from build123d import *

# Parameters (mm, degrees)
CROQUIS1_W              = 3
CROQUIS1_H              = 15
CROQUIS1_R              = 1.25
SALIENTE_EXTRUIR1_DEPTH = 3
CROQUIS2_W              = 3
CROQUIS2_H              = 15
CORTAR_EXTRUIR1_DEPTH   = 3
CROQUIS3_W              = 10
CROQUIS3_H              = 3
SALIENTE_EXTRUIR2_DEPTH = 3
CROQUIS4_W              = 12
CROQUIS4_H              = 18.363871442
CORTAR_EXTRUIR2_DEPTH   = 3


with BuildPart() as part:
    # Croquis1 → Saliente-Extruir1 (new body)
    with BuildSketch(Plane.XY):
        with BuildLine():
            Line((103, 21.25), (103, 30))
            Line((103, 30), (69.2, 30))
            Line((69.2, 30), (69.2, 22))
            Line((69.2, 22), (71.35, 22))
            Line((71.35, 22), (71.35, 19))
            Line((71.35, 19), (69.2, 19))
            Line((69.2, 19), (69.2, 15))
            Line((69.2, 15), (66.5, 15))
            Line((66.5, 15), (66.5, 19))
            Line((66.5, 19), (64.35, 19))
            Line((64.35, 19), (64.35, 22))
            Line((64.35, 22), (66.5, 22))
            Line((66.5, 22), (66.5, 30))
            Line((66.5, 30), (36.5, 30))
            Line((36.5, 30), (36.5, 22))
            Line((36.5, 22), (38.65, 22))
            Line((38.65, 22), (38.65, 19))
            Line((38.65, 19), (36.5, 19))
            Line((36.5, 19), (36.5, 15))
            Line((36.5, 15), (33.8, 15))
            Line((33.8, 15), (33.8, 19))
            Line((33.8, 19), (31.65, 19))
            Line((31.65, 19), (31.65, 22))
            Line((31.65, 22), (33.8, 22))
            Line((33.8, 22), (33.8, 30))
            Line((33.8, 30), (0, 30))
            Line((0, 30), (0, 21.25))
            Line((0, 21.25), (1.5, 21.25))
            ThreePointArc((1.5, 21.25), (2.75, 20), (1.5, 18.75))
            Line((1.5, 18.75), (0, 18.75))
            Line((0, 18.75), (0, 0))
            Line((0, 0), (0, -10))
            Line((0, -10), (3, -10))
            Line((3, -10), (3, -20))
            Line((3, -20), (0, -20))
            Line((0, -20), (0, -35))
            Line((0, -35), (3, -35))
            Line((3, -35), (3, -50))
            Line((3, -50), (0, -50))
            Line((0, -50), (0, -65))
            Line((0, -65), (3, -65))
            Line((3, -65), (3, -80))
            Line((3, -80), (0, -80))
            Line((0, -80), (0, -92))
            Line((0, -92), (6.427876097, -99.660444431))
            Line((6.427876097, -99.660444431), (8.726009426, -97.732081602))
            Line((8.726009426, -97.732081602), (15.153885523, -105.392526033))
            Line((15.153885523, -105.392526033), (12.855752194, -107.320888862))
            Line((12.855752194, -107.320888862), (19.283628291, -114.981333294))
            Line((19.283628291, -114.981333294), (80.56718374, -63.558324519))
            Line((80.56718374, -63.558324519), (80.56718374, -50))
            Line((80.56718374, -50), (77.56718374, -50))
            Line((77.56718374, -50), (77.56718374, -35))
            Line((77.56718374, -35), (103, -35))
            Line((103, -35), (103, -16.25))
            Line((103, -16.25), (101.5, -16.25))
            ThreePointArc((101.5, -16.25), (100.25, -15), (101.5, -13.75))
            Line((101.5, -13.75), (103, -13.75))
            Line((103, -13.75), (103, 18.75))
            Line((103, 18.75), (101.5, 18.75))
            ThreePointArc((101.5, 18.75), (100.25, 20), (101.5, 21.25))
            Line((101.5, 21.25), (103, 21.25))
        make_face()
        with Locations((79.06718374, 2.5)):
            Rectangle(CROQUIS1_W, CROQUIS1_H, mode=Mode.SUBTRACT)
        with Locations((79.06718374, 20)):
            Circle(CROQUIS1_R, mode=Mode.SUBTRACT)
    extrude(amount=SALIENTE_EXTRUIR1_DEPTH)

    # Croquis2 → Cortar-Extruir1 (cut)
    with BuildSketch(Plane(origin=(103, 0, 0), x_dir=(0, 0, -1), z_dir=(1, 0, 0))):
        with Locations((-1.5, 2.5)):
            Rectangle(CROQUIS2_W, CROQUIS2_H)
    extrude(amount=-CORTAR_EXTRUIR1_DEPTH, mode=Mode.SUBTRACT)

    # Croquis3 → Saliente-Extruir2 (add)
    with BuildSketch(Plane.XY.offset(3)):
        with Locations((15, 31.5)):
            Rectangle(CROQUIS3_W, CROQUIS3_H)
        with Locations((88, 31.5)):
            Rectangle(CROQUIS3_W, CROQUIS3_H)
    extrude(amount=-SALIENTE_EXTRUIR2_DEPTH)

    # Croquis4 → Cortar-Extruir2 (cut)
    with BuildSketch(Plane.XY.offset(3)):
        with Locations((90.304087079, -4.709619469)):
            Rectangle(CROQUIS4_W, CROQUIS4_H)
    extrude(amount=-CORTAR_EXTRUIR2_DEPTH, mode=Mode.SUBTRACT)


solid = part.part
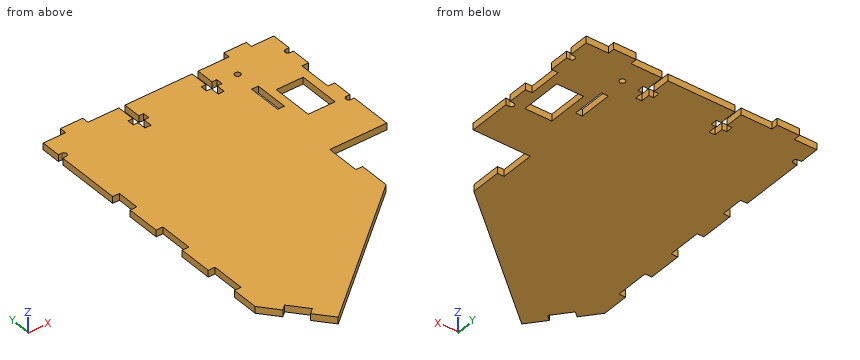
For this review, take the finished solid that the model builds, in its own axes (mm). Round coordinates to 2 decimals unless told otherwise and drop trailing zeros. Loops run counter-clockwise (first coordinate to the right, second up) from the corner with the lowest first, then second, coordinate; pieces in that order, holes last. Notation, with made-up numbers: (-25.75, 81) - (-8.75, 81) arc R9 cw to (-8.75, 87) - close; hole circle Ø7 at (-19.5, 33). An arc over 180 degrees is marked (long way). Use one line per item in the form item = value.
Item 1: Consider section C-C on z = 1.3. State how many separate pieces and enclosed holes the cut face has, then the cut area to 3 significant figures.
Answers:
separate_pieces = 1
enclosed_holes = 3
area = 10,800 mm^2
Item 2: Clearance check with flat-ended pins moving along their axes: P1, Ø1.5, axis at x = 36, y = 6.5, coming from the -Z side; P2, Ø1.5, axis at y = -59.5, z = 1, coming from the +X side; P3, Ø1.7, axis at x = 65.5, z = 1, coming from the +Y side; P4, Ø1.5, axis at y = -39.5, z = 2, coming from the +X side. State where each tip first meets the part, or that it passes through.
Answers:
P1 = 0
P2 = 80.57
P3 = 30
P4 = 77.57
Item 3: For line 1 (X direction, y = 5, z = 0.4); line 2 (Y direction, x = 14, z = 1.35); line 3 (X direction, y = -42.5, z = 1.8), list the stretches that pass through material, from the lowest coordinate up.
Answers:
line_1 = 0 to 77.57, 80.57 to 100
line_2 = -108.68 to -106.36, -104.02 to 33
line_3 = 3 to 77.57
Item 4: Consider section B-B on y = -46. Write out the cut boundary in (x, z).
Answers:
outline = (3, 0) - (77.57, 0) - (77.57, 3) - (3, 3) - close
Item 5: Consider section A-A on x = 90. Write out the cut boundary in (y, z).
Answers:
outline = (-35, 0) - (-13.89, 0) - (-13.89, 3) - (-35, 3) - close; (4.47, 0) - (33, 0) - (33, 3) - (4.47, 3) - close
Item 6: Consider section D-D on x = 28. Write out the cut boundary in (y, z), then the cut area to 3 significant figures.
Answers:
outline = (-107.67, 0) - (30, 0) - (30, 3) - (-107.67, 3) - close
area = 413 mm^2
